Print and shaded views of the part. All mm, measured from the part's lowest x, y and z. A direction names the side the tool comes from. Give positions to 0.01 mm unless a question says otherwise; leave off trailing zeros. Write each loop counter-clockwise with the first axis right and the second up, starting at its lowest first coordinate (ties: lowest second). Pieces come first, ordered by that corner, then holes. Notation, with made-up numbers: (-16, -26) -> (21, -26) arc R27 cw to (21, 9) -> close; hole circle Ø8 at (37.25, -13). An arc over 180 degrees is marked (long way). Put each result on its own line as item: value.
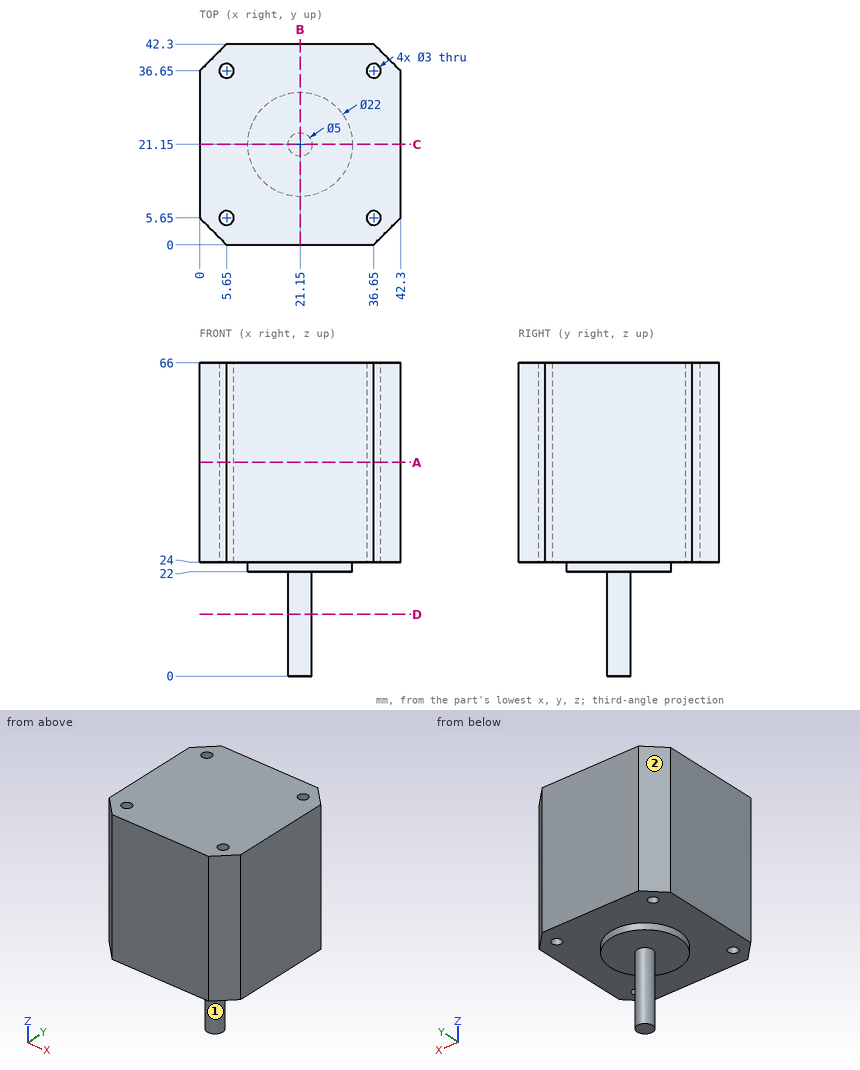
1) Slice it at A-A (z = 45). Write the cut outline in (x, y).
Filled sheet:
outline: (0, 5.65) -> (5.65, 0) -> (36.65, 0) -> (42.3, 5.65) -> (42.3, 36.65) -> (36.65, 42.3) -> (5.65, 42.3) -> (0, 36.65) -> close; hole circle Ø3 at (5.65, 5.65); hole circle Ø3 at (5.65, 36.65); hole circle Ø3 at (36.65, 5.65); hole circle Ø3 at (36.65, 36.65)
2) Slice it at D-D (z = 13). Write the cut outline in (x, y).
Filled sheet:
outline: circle Ø5 at (21.15, 21.15)
3) Wall check: L1, parallel to Y at x = 36.65, z = 33; L2, parallel to Y at x = 5, z = 42; L3, parallel to X at y = 37, z = 43.5. Give the ranges that are in metal, low to high.
Filled sheet:
L1: 0 to 4.15, 7.15 to 35.15, 38.15 to 42.3
L2: 0.65 to 4.3, 7 to 35.3, 38 to 41.65
L3: 0.35 to 4.19, 7.11 to 35.19, 38.11 to 41.95
4) Pin check, flat tips, straight feed: pin 1 (4 mm diameter, centred on x = 18, z = 11.5, fed in from -Y); pin 2 (5 mm diameter, centred on x = 36.65, y = 5.65, fed in from -Z); pin 3 (1.8 mm diameter, centred on x = 36.65, y = 36.65, fed in from +Z); pin 4 (8 mm diameter, centred on x = 25, z = 13.5, fed in from -Y). Stop position of each tip, or through.
Filled sheet:
pin 1: y = 18.93
pin 2: z = 24
pin 3: through
pin 4: y = 18.65
5) Slice it at B-B (x = 21.15). Write the cut outline in (y, z).
Filled sheet:
outline: (0, 24) -> (10.15, 24) -> (10.15, 22) -> (18.65, 22) -> (18.65, 0) -> (23.65, 0) -> (23.65, 22) -> (32.15, 22) -> (32.15, 24) -> (42.3, 24) -> (42.3, 66) -> (0, 66) -> close
6) Tool access for the marked faces 1 and 2: list every direction of +Z, -Z, +X, -X, +Y, -Y with a clear straight run to the whole face (end or side of a thin tool).
Filled sheet:
face 1: -Z
face 2: +Z, -Z, -X, +Y
